Here's how the part is built. I have some questions about the finished solid (model axes, mm). A direction names the side the tool comes from. Coordinates: 2 decimals unless noted, no trailing zeros. Loops run counter-clockwise (first coordinate to the right, second up) from the corner with the lowest first, then second, coordinate; pieces in that order, holes last. Notation, with made-up numbers: (46.25, 86.25) -> (102.25, 86.25) arc R20 cw to (102.25, 109.25) -> close; hole circle Ø10 at (83, 33). An arc over 180 degrees is marked (long way). Answer as a JSON object with one key per item and string values. Group by question number.
1) If we mould it in two halves opening along Y, with no side actions, what happens to faces 1 (the flat face through (-1, 1, -8)), 2 (the flat face through (-1, -20, -7)), 3 (the flat face through (-1, -18, -10))? For each: +Y half, -Y half, draft (parallel to the pull), parting line (faces both ways), or undercut.
2) I want a section at D-D (z = -14). Write out the boundary of the cut face in (x, y), then the cut area to 3 significant figures.
3) I want a section at C-C (x = -20). Write out the boundary of the cut face in (y, z).
4) I'm going to push flat-ended pins straight in: pin 1 (13.5 mm diameter, centred on x = 34, y = 10, fed in from -Z); pin 2 (7 mm diameter, centred on x = 20.4, y = 10, fed in from -Z); pin 3 (1.1 mm diameter, centred on x = 8.5, y = -18.5, fed in from -Z); pin 4 (2.5 mm diameter, centred on x = -10.5, z = -10.5, fed in from +Y). Where does each tip first touch, or does it pass through?
5) I want a section at A-A (y = 10). Write out the boundary of the cut face in (x, z).
6) Which directions (+Z, -Z, +X, -X, +Y, -Y) give clear straight access to the entire face, cutting with the end or side of a thin tool? Please do faces 4 (the flat face through (-1, -23, -10)), 5 (the flat face through (40, -10, -5)).
7) I want a section at B-B (x = 20.4). Write out the boundary of the cut face in (y, z), then the cut area to 3 significant figures.
8) I need wall thicknesses on probe 1 along Y at (x, z) = (34, -5.5); probe 2 along Y at (x, z) = (-6.5, -1.75); probe 3 along Y at (x, z) = (21.5, -10.5). Which ranges of each line are inside material? Lowest first, please. Write a range as [from, to].
```python
from build123d import *

# Parameters (mm, degrees)
F0_W     = 80
F0_H     = 40
F1_DEPTH = 8
F0_H_2   = 3
F2_DEPTH = 2.5
F0_H_3   = 3.5
F3_DEPTH = 20
F5_D     = 8.5
F6_R     = 2
F7_R     = 5
F8_W     = 80
F8_H     = 2
F9_DEPTH = 5
F10_SIZE = 1


with BuildPart() as f1:
    # F0 (on Top) → F1 (new body)
    with BuildSketch(Plane.XY):
        Rectangle(F0_W, F0_H)
    extrude(amount=-F1_DEPTH)

    # F0 (on Top) → F2 (join)
    with BuildSketch(Plane.XY):
        with Locations((0, -21.5)):
            Rectangle(F0_W, F0_H_2)
    extrude(amount=-F2_DEPTH)

    # F0 (on Top) → F3 (join)
    with BuildSketch(Plane.XY):
        with Locations((0, -24.75)):
            Rectangle(F0_W, F0_H_3)
    extrude(amount=-F3_DEPTH)

    # F5 (through all)
    with Locations(Plane.XY):
        with Locations((-34, 10), (34, 10), (6.8, 10), (20.4, 10), (-20.4, 10), (-6.8, 10)):
            Hole(F5_D / 2)

    # F6
    f6_edges = [f1.edges().sort_by_distance(p)[0] for p in [
        (0, -23, -20),
    ]]
    fillet(f6_edges, radius=F6_R)

    # F7
    f7_edges = [f1.edges().sort_by_distance(p)[0] for p in [
        (40, 20, -4),
        (-40, 20, -4),
    ]]
    fillet(f7_edges, radius=F7_R)

    # F8 (on face) → F9 (join)
    with BuildSketch(Plane(origin=(0, 0, -8), x_dir=(1, 0, 0), z_dir=(0, 0, -1))):
        with Locations((0, 19)):
            Rectangle(F8_W, F8_H)
    extrude(amount=F9_DEPTH)

    # F10
    f10_edges = [f1.edges().sort_by_distance(p)[0] for p in [
        (0, -20, -13),
    ]]
    chamfer(f10_edges, length=F10_SIZE)


solid = f1.part
```
Determined:
{
 "1": {"face 1": "draft", "face 2": "undercut", "face 3": "+Y half"},
 "2": {"outline": "(-40, -26.5) -> (40, -26.5) -> (40, -23) -> (-40, -23) -> close", "area": "280 mm^2"},
 "3": {"outline": "(-26.5, -20) -> (-25, -20) arc R2 ccw to (-23, -18) -> (-23, -2.5) -> (-20, -2.5) -> (-20, -12) -> (-19, -13) -> (-18, -13) -> (-18, -8) -> (5.77, -8) -> (5.77, 0) -> (-26.5, 0) -> close; (14.23, -8) -> (20, -8) -> (20, 0) -> (14.23, 0) -> close"},
 "4": {"pin 1": "z = -8", "pin 2": "through", "pin 3": "z = -13", "pin 4": "y = -18"},
 "5": {"outline": "(-40, -8) -> (-38.25, -8) -> (-38.25, 0) -> (-40, 0) -> close; (-29.75, -8) -> (-24.65, -8) -> (-24.65, 0) -> (-29.75, 0) -> close; (-16.15, -8) -> (-11.05, -8) -> (-11.05, 0) -> (-16.15, 0) -> close; (-2.55, -8) -> (2.55, -8) -> (2.55, 0) -> (-2.55, 0) -> close; (11.05, -8) -> (16.15, -8) -> (16.15, 0) -> (11.05, 0) -> close; (24.65, -8) -> (29.75, -8) -> (29.75, 0) -> (24.65, 0) -> close; (38.25, -8) -> (40, -8) -> (40, 0) -> (38.25, 0) -> close"},
 "6": {"face 4": "-Z, +X, -X", "face 5": "+Z, -Z, +X, +Y, -Y"},
 "7": {"outline": "(-26.5, -20) -> (-25, -20) arc R2 ccw to (-23, -18) -> (-23, -2.5) -> (-20, -2.5) -> (-20, -12) -> (-19, -13) -> (-18, -13) -> (-18, -8) -> (5.75, -8) -> (5.75, 0) -> (-26.5, 0) -> close; (14.25, -8) -> (20, -8) -> (20, 0) -> (14.25, 0) -> close", "area": "338 mm^2"},
 "8": {"probe 1": "[-26.5, -23], [-20, 5.75], [14.25, 20]", "probe 2": "[-26.5, 5.76], [14.24, 20]", "probe 3": "[-26.5, -23], [-20, -18]"}
}
